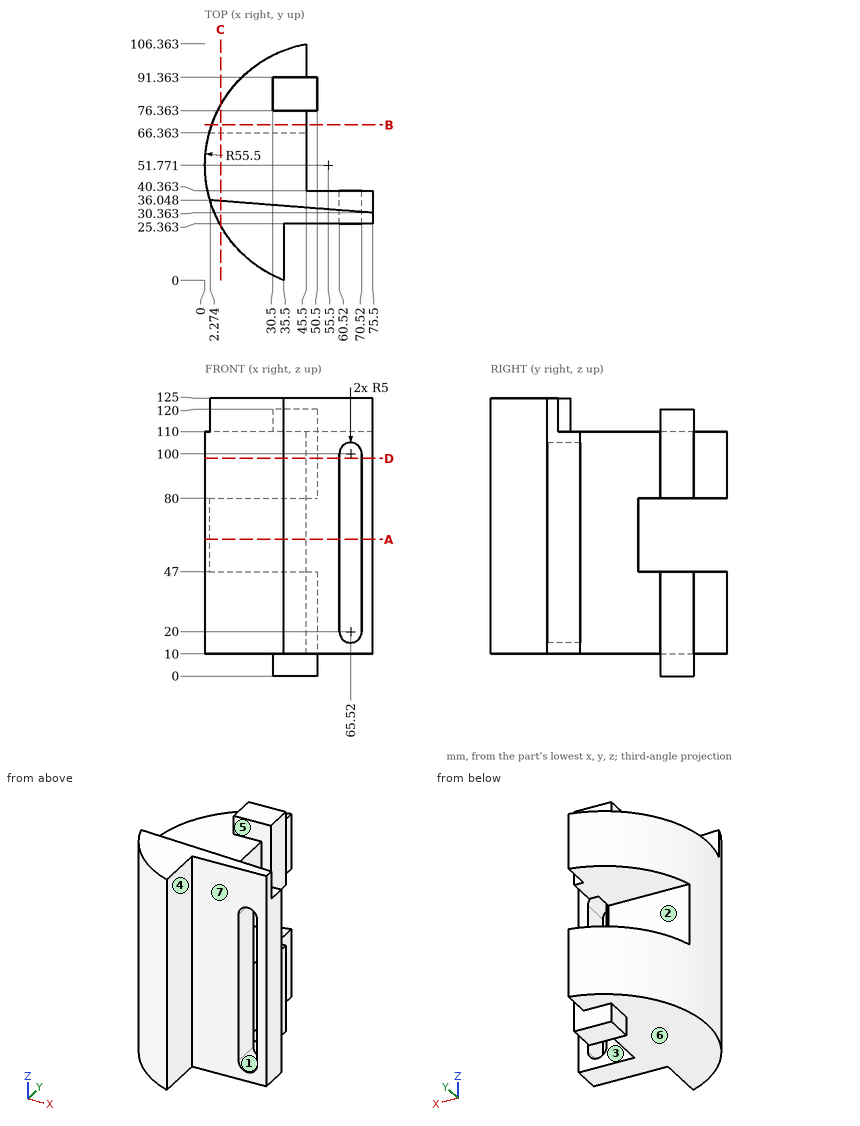
Geometry check sheet. Reference: drawing and pictorial views, mm from the part's lowest x, y, z. A direction names the side the tool comes from. Give positions to 0.01 mm unless a question says otherwise; leave off trailing zeros. Order: outer loops, then holes, each group sorted by start corner. A loop starts at its lowest first (then second) coordinate and runs counter-clockwise, first axis right, second up. Notation, with made-up numbers: M 70.25,73.5 L 111.25,73.5 A20 cw 111.25,95.5 Z; hole C 52,79.25 d2. An arc over 180 degrees is marked long. Answer as a JSON object with one key per item and string values. Group by question number.
1) Cross-section at D-D (z = 98). Enter the section's corners in (x, y).
2) Depth check by flat-ended pin: pin 1 Ø16 at (x, z) = (38.5, 19.5) entering from +Y; pin 2 Ø8 at (y, z) = (12, 75) entering from -X (1 decimal); pin 3 Ø4.5 at (y, z) = (83, 29.5) entering from +X; pin 4 Ø2 at (x, y) = (37, 84.5) entering from -Z. Enter the tip coordinate at first touch or a pass-through.
3) Scan lines: line 1 along Z through (x, y) = (8.5, 71); line 2 along Y through (x, z) = (49.5, 34); line 3 along Y through (x, z) = (51.5, 75). Record each from-to range of solid material in increasing order. Write a range as [from, to].
4) Cross-section at B-B (y = 70). Enter the section's corners in (x, z), then the cut area to 3 significant figures.
5) Cross-section at A-A (z = 61.5). Enter the section's corners in (x, y).
6) Cross-section at C-C (x = 7). Enter the section's corners in (y, z), then the cut area to 3 significant figures.
7) Mould release check, pull along Y, two halves, no side actions. Record for the marked faces 5, 6 and 7: released by +Y, released by -Y, zero draft, split by the parting line, or undercut.
8) Access from +Z, -Z, +X, -X, +Y, -Y to the whole of each face (thin tool, end or side, straight path). Record for the marked faces 1, 2, 3 and 4.
Result sheet:
{
 "1": {"outline": "M 35.5,0 L 35.5,25.36 L 60.52,25.36 L 60.52,40.36 L 45.5,40.36 L 45.5,76.36 L 50.5,76.36 L 50.5,91.36 L 45.5,91.36 L 45.5,106.36 A55.5 ccw Z; M 70.52,25.36 L 75.5,25.36 L 75.5,40.36 L 70.52,40.36 Z"},
 "2": {"pin 1": "stops at y = 106.36", "pin 2": "stops at x = 13.1", "pin 3": "stops at x = 50.5", "pin 4": "stops at z = 0"},
 "3": {"line 1": "z = [10, 47], [80, 110]", "line 2": "y = [25.36, 40.36], [76.36, 91.36]", "line 3": "y = [25.36, 40.36]"},
 "4": {"outline": "M 3.08,10 L 45.5,10 L 45.5,47 L 3.08,47 Z; M 3.08,80 L 45.5,80 L 45.5,110 L 3.08,110 Z", "area": "2,840 mm2"},
 "5": {"outline": "M 1.95,66.36 A55.5 ccw 35.5,0 L 35.5,25.36 L 60.52,25.36 L 60.52,40.36 L 45.5,40.36 L 45.5,66.36 Z; M 70.52,25.36 L 75.5,25.36 L 75.5,40.36 L 70.52,40.36 Z"},
 "6": {"outline": "M 24.79,10 L 78.75,10 L 78.75,47 L 66.36,47 L 66.36,80 L 78.75,80 L 78.75,110 L 35.68,110 L 35.68,125 L 24.79,125 Z", "area": "5,150 mm2"},
 "7": {"face 5": "undercut", "face 6": "zero draft", "face 7": "released by -Y"},
 "8": {"face 1": "+Y, -Y", "face 2": "+X, -X, +Y", "face 3": "+Z, -Z, +X", "face 4": "+Z, -Z, +X, -Y"}
}
